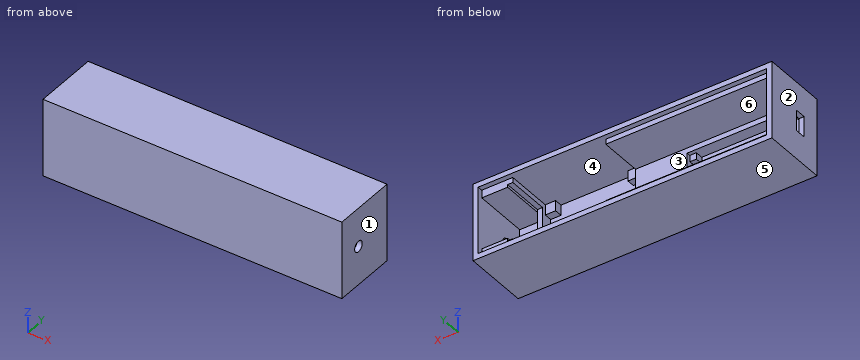
```python
from build123d import *

# Parameters (mm, degrees)
ESQUISSE1_W             = 115.7
ESQUISSE1_H             = 30
ESQUISSE1_W_2           = 36
ESQUISSE1_H_2           = 26
ESQUISSE1_W_3           = 43.7
ESQUISSE1_H_3           = 18.1
ESQUISSE1_W_4           = 10
ESQUISSE1_H_4           = 20
BOSS_EXTRU_1_DEPTH      = 21
ESQUISSE2_W             = 115.7
ESQUISSE2_H             = 30
BOSS_EXTRU_2_DEPTH      = 2
ESQUISSE3_W             = 2.5
ESQUISSE3_H             = 2.5
BOSS_EXTRU_3_DEPTH      = 3
ESQUISSE4_W             = 4
ESQUISSE4_H             = 4
BOSS_EXTRU_4_DEPTH      = 3
ESQUISSE5_W             = 8
ESQUISSE5_H             = 4.2
ENL_V_MAT_EXTRU_1_DEPTH = 2
ESQUISSE7_W             = 101.7
ESQUISSE7_H             = 22.1
ENL_V_MAT_EXTRU_2_DEPTH = 16.5
ESQUISSE8_R             = 2.1
ENL_V_MAT_EXTRU_3_DEPTH = 2
ESQUISSE9_W             = 115.7
ESQUISSE9_H             = 30
ESQUISSE9_W_2           = 111.7
ESQUISSE9_H_2           = 26
BOSS_EXTRU_5_DEPTH      = 2


with BuildPart() as part:
    # Esquisse1 → Boss.-Extru.1 (new body)
    with BuildSketch(Plane(origin=(0, 0, 0), x_dir=(1, 0, 0), z_dir=(0, 1, 0))):
        with Locations((-7.85, 13)):
            Rectangle(ESQUISSE1_W, ESQUISSE1_H)
        with Locations((18, 13)):
            Rectangle(ESQUISSE1_W_2, ESQUISSE1_H_2, mode=Mode.SUBTRACT)
        with Locations((-41.85, 13)):
            Rectangle(ESQUISSE1_W_3, ESQUISSE1_H_3, mode=Mode.SUBTRACT)
        with Locations((43, 13)):
            Rectangle(ESQUISSE1_W_4, ESQUISSE1_H_4, mode=Mode.SUBTRACT)
    extrude(amount=BOSS_EXTRU_1_DEPTH)

    # Esquisse2 → Boss.-Extru.2 (add)
    with BuildSketch(Plane(origin=(0, 0, 0), x_dir=(-1, 0, 0), z_dir=(0, -1, 0))):
        with Locations((7.85, 13)):
            Rectangle(ESQUISSE2_W, ESQUISSE2_H)
    extrude(amount=BOSS_EXTRU_2_DEPTH)

    # Esquisse3 → Boss.-Extru.3 (add)
    with BuildSketch(Plane(origin=(0, 0, 0), x_dir=(1, 0, 0), z_dir=(0, 1, 0))):
        with Locations((-62.45, 20.8)):
            Rectangle(ESQUISSE3_W, ESQUISSE3_H)
        with Locations((-21.25, 20.8)):
            Rectangle(ESQUISSE3_W, ESQUISSE3_H)
        with Locations((-21.25, 5.2)):
            Rectangle(ESQUISSE3_W, ESQUISSE3_H)
        with Locations((-62.45, 5.2)):
            Rectangle(ESQUISSE3_W, ESQUISSE3_H)
    extrude(amount=BOSS_EXTRU_3_DEPTH)

    # Esquisse4 → Boss.-Extru.4 (add)
    with BuildSketch(Plane(origin=(0, 0, 0), x_dir=(1, 0, 0), z_dir=(0, 1, 0))):
        with Locations((2, 24)):
            Rectangle(ESQUISSE4_W, ESQUISSE4_H)
        with Locations((34, 24)):
            Rectangle(ESQUISSE4_W, ESQUISSE4_H)
        with Locations((34, 2)):
            Rectangle(ESQUISSE4_W, ESQUISSE4_H)
        with Locations((2, 2)):
            Rectangle(ESQUISSE4_W, ESQUISSE4_H)
    extrude(amount=BOSS_EXTRU_4_DEPTH)

    # Esquisse5 → Enlèv. mat.-Extru.1 (cut)
    with BuildSketch(Plane(origin=(-63.7, 0, 0), x_dir=(0, 0, -1), z_dir=(1, 0, 0))):
        with Locations((13, 7.2)):
            Rectangle(ESQUISSE5_W, ESQUISSE5_H)
    extrude(amount=-ENL_V_MAT_EXTRU_1_DEPTH, mode=Mode.SUBTRACT)

    # Esquisse7 → Enlèv. mat.-Extru.2 (cut)
    with BuildSketch(Plane(origin=(0, 4.5, 0), x_dir=(1, 0, 0), z_dir=(0, 1, 0))):
        with Locations((-12.85, 13)):
            Rectangle(ESQUISSE7_W, ESQUISSE7_H)
    extrude(amount=ENL_V_MAT_EXTRU_2_DEPTH, mode=Mode.SUBTRACT)

    # Esquisse8 → Enlèv. mat.-Extru.3 (cut)
    with BuildSketch(Plane.ZY.offset(-48)):
        with Locations((-13, 7.2)):
            Circle(ESQUISSE8_R)
    extrude(amount=-ENL_V_MAT_EXTRU_3_DEPTH, mode=Mode.SUBTRACT)

    # Esquisse9 → Boss.-Extru.5 (add)
    with BuildSketch(Plane(origin=(0, 21, 0), x_dir=(1, 0, 0), z_dir=(0, 1, 0))):
        with Locations((-7.85, 13)):
            Rectangle(ESQUISSE9_W, ESQUISSE9_H)
        with Locations((-7.85, 13)):
            Rectangle(ESQUISSE9_W_2, ESQUISSE9_H_2, mode=Mode.SUBTRACT)
    extrude(amount=BOSS_EXTRU_5_DEPTH)


solid = part.part
```
For this review, take the finished solid that the model builds, in its own axes (mm). Face numbers are marked on the shaded views. A direction names the side the tool comes from. Coordinates: 2 decimals unless noted, no trailing zeros. Loops run counter-clockwise (first coordinate to the right, second up) from the corner with the lowest first, then second, coordinate; pieces in that order, holes last.
1. Add section D-D, the plane x = 13.5. Give the boundary of the cut face in (y, z), then the cut area to 3 significant figures.
2. Add section B-B, the plane y = 13.5. Give the boundary of the cut face in (x, z).
3. Insertion check: P1, Ø8, axis at x = 0, z = -1.5, coming from the +Y side; P2, Ø6, axis at x = -51, z = -20.5, coming from the +Y side; P3, Ø2, axis at x = -62.5, z = -21, coming from the +Y side; P4, Ø1, axis at x = 32, z = -8, coming from the +Y side. Each pin has a flat end and moves straight along its axis. Give the tip position at first contact, or say it passes through.
4. For line 1 (X direction, y = 1.75, z = -8); line 2 (X direction, y = 5.5, z = -5.25); line 3 (X direction, y = 5, z = -23.75), list the stretches that pass through material, from the lowest coordinate up.
5. For the marked faces 5 and 6, list the 3-axis set-ups (+Z, -Z, +X, -X, +Y, -Y) from which the entire face can be reached by the end or side of a thin tool; tool diameter is ignored.
6. Add section C-C, the plane y = 7.2. Give the boundary of the cut face in (x, z), then the cut area to 3 significant figures.
7. Mouldability with a two-part tool opening along X and no side actions: class the marked faces 1, 2, 3 and 4 as +X half, -X half, draft (parallel to the pull), parting line (faces both ways), or undercut.
8. Add section A-A, the plane z = -13. Give the boundary of the cut face in (x, y), then the cut area to 3 significant figures.
Result:
1. outline: (-2, -28) - (23, -28) - (23, -26) - (0, -26) - (0, 0) - (23, 0) - (23, 2) - (-2, 2) - close
1. area: 152 mm2
2. outline: (-65.7, -28) - (50, -28) - (50, 2) - (-65.7, 2) - close; hole (-63.7, -24.05) - (0, -24.05) - (0, -26) - (36, -26) - (36, -24.05) - (38, -24.05) - (38, -23) - (48, -23) - (48, -3) - (38, -3) - (38, -1.95) - (36, -1.95) - (36, 0) - (0, 0) - (0, -1.95) - (-63.7, -1.95) - close
3. P1: stops at y = 23
3. P2: stops at y = 4.5
3. P3: stops at y = 3
3. P4: stops at y = 0
4. line 1: x = -65.7 to -63.7, -20 to 0, 36 to 38, 48 to 50
4. line 2: x = -65.7 to -63.7, 48 to 50
4. line 3: x = -65.7 to -63.7, 38 to 50
5. face 5: -Z, +X, -X, +Y, -Y
5. face 6: +Y
6. outline: (-65.7, -28) - (50, -28) - (50, -15.1) - (48, -15.1) - (48, -23) - (38, -23) - (38, -24.05) - (36, -24.05) - (36, -26) - (0, -26) - (0, -24.05) - (-63.7, -24.05) - (-63.7, -17) - (-65.7, -17) - close; (-65.7, -9) - (-63.7, -9) - (-63.7, -1.95) - (0, -1.95) - (0, 0) - (36, 0) - (36, -1.95) - (38, -1.95) - (38, -3) - (48, -3) - (48, -10.9) - (50, -10.9) - (50, 2) - (-65.7, 2) - close
6. area: 859 mm2
7. face 1: +X half
7. face 2: -X half
7. face 3: undercut
7. face 4: undercut
8. outline: (-65.7, -2) - (50, -2) - (50, 5.1) - (48, 5.1) - (48, 0) - (38, 0) - (38, 4.5) - (36, 4.5) - (36, 0) - (0, 0) - (0, 4.5) - (-20, 4.5) - (-20, 0) - (-63.7, 0) - (-63.7, 5.1) - (-65.7, 5.1) - close; (-65.7, 9.3) - (-63.7, 9.3) - (-63.7, 23) - (-65.7, 23) - close; (48, 9.3) - (50, 9.3) - (50, 23) - (48, 23) - close
8. area: 406 mm2
